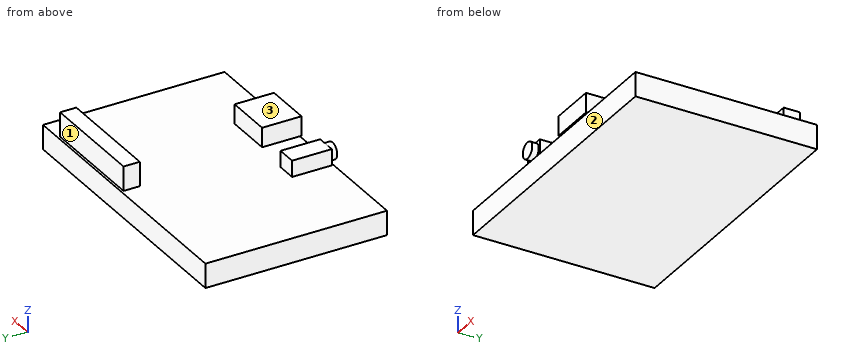
Autodesk Inventor part; units mm, degrees
ref_plane "YZ Plane" through (0, 0, 0) normal (1, 0, 0) x (0, 1, 0)
ref_plane "XZ Plane" through (0, 0, 0) normal (0, 1, 0) x (-1, 0, 0)
ref_plane "XY Plane" through (0, 0, 0) normal (0, 0, 1) x (1, 0, 0)
sketch "Sketch1" plane through (0, 0, 0) normal (0, 0, 1) x (1, 0, 0)
  line L0 (0, 0) -> (85.75, 0)
  line L1 (85.75, 0) -> (85.75, 56)
  line L2 (85.75, 56) -> (0, 56)
  line L3 (0, 56) -> (0, 0)
  dimension "d0" = 85.75
  dimension "d1" = 56
extrude "Extrusion1" add sketch "Sketch1" along normal blind 7.5
sketch "Sketch3" plane through (0, 0, 7.5) normal (0, 0, 1) x (1, 0, 0)
  line L0 (78, 55.25) -> (44.5, 55.25)
  line L1 (44.5, 55.25) -> (44.5, 50.25)
  line L2 (44.5, 50.25) -> (78, 50.25)
  line L3 (78, 50.25) -> (78, 55.25)
  line L4 (85.75, 56) -> (0, 56)
  line L5 (85.75, 0) -> (85.75, 56)
  point P0 (0, 0)
  dimension "d19" = 33.5
  dimension "d20" = 5
  dimension "d21" = 0.75
  dimension "d22" = 7.75
extrude "Extrusion3" add sketch "Sketch3" along normal blind 7.5
sketch "Sketch4" plane through (0, 0, 7.5) normal (0, 0, 1) x (1, 0, 0)
  line L0 (46, 11.65) -> (60.5, 11.65)
  line L1 (60.5, 11.65) -> (60.5, -0.5)
  line L2 (60.5, -0.5) -> (46, -0.5)
  line L3 (46, -0.5) -> (46, 11.65)
  line L4 (0, 0) -> (85.75, 0)
  line L5 (85.75, 0) -> (85.75, 56)
  dimension "d25" = 14.5
  dimension "d26" = 12.15
  dimension "d28" = 0.5
  dimension "d29" = 25.25
extrude "Extrusion4" add sketch "Sketch4" along normal blind 6
sketch "Sketch5" plane through (0, 0, 7.5) normal (0, 0, 1) x (1, 0, 0)
  line L0 (28.3, 12.75) -> (34.4, 12.75)
  line L1 (34.4, 12.75) -> (34.4, 0.5)
  line L2 (34.4, 0.5) -> (28.3, 0.5)
  line L3 (28.3, 0.5) -> (28.3, 12.75)
  line L4 (0, 0) -> (46, 0)
  line L5 (0, 56) -> (0, 0)
  dimension "d32" = 12.25
  dimension "d33" = 6.1
  dimension "d35" = 28.3
  dimension "d36" = 0.5
extrude "Extrusion5" add sketch "Sketch5" along normal blind 5
sketch "Sketch6" plane through (28.3, 0.5, 7.5) normal (0, -1, 0) x (1, 0, 0)
  line L0 (6.1, 5) -> (0, 5)
  line L1 (3.05, 5) -> (3.05, 2.5)
  circle A0 centre (3.05, 2.5) radius 2.5
  point P0 (-28.3, -7.5)
  dimension "d39" = 2.5
  dimension "d40" = 5
extrude "Extrusion6" add sketch "Sketch6" along normal blind 2
properties part number "RaspberryPi3_Screen"
Verification items for the finished model (mm, model axes). Face numbers are marked on the shaded views. A direction names the side the tool comes from. Coordinates: 2 decimals unless noted, no trailing zeros. Write each loop counter-clockwise with the first axis right and the second up, starting at its lowest first coordinate (ties: lowest second). Pieces come first, ordered by that corner, then holes. Notation, with made-up numbers: M -10.5,51.25 L 5.5,51.25 A21 cw 5.5,79.25 Z; hole C -2,38.5 d1. An arc over 180 degrees is marked long. Use a Markdown table: item, result.
Q1. Sectioned sample at A-A, the plane y = 3.5. Record the boundary of the cut face in (x, z).
Reply:
| item | result |
|---|---|
| outline | M 0,0 L 85.75,0 L 85.75,7.5 L 60.5,7.5 L 60.5,13.5 L 46,13.5 L 46,7.5 L 34.4,7.5 L 34.4,12.5 L 28.3,12.5 L 28.3,7.5 L 0,7.5 Z |
Q2. Sectioned sample at C-C, the plane z = 6.5. Record the boundary of the cut face in (x, y), plus the area to 3 significant figures.
Reply:
| item | result |
|---|---|
| outline | M 0,0 L 85.75,0 L 85.75,56 L 0,56 Z |
| area | 4,800 mm² |
Q3. Go/stop test with flat-tipped pins: P1, Ø5.5, axis at x = 30.5, z = 10.5, coming from the +Y side; P2, Ø2, axis at x = 54.5, z = 12, coming from the +Y side; P3, Ø2, axis at x = 55.5, y = 31, coming from the +Z side; P4, Ø8, axis at x = 76.5, y = 28, coming from the -Z side. Record where each tip stops, or that it passes through.
Reply:
| item | result |
|---|---|
| P1 | stops at y = 12.75 |
| P2 | stops at y = 55.25 |
| P3 | stops at z = 7.5 |
| P4 | stops at z = 0 |
Q4. Sectioned sample at B-B, the plane x = 57. Record the boundary of the cut face in (y, z), plus the area to 3 significant figures.
Reply:
| item | result |
|---|---|
| outline | M -0.5,7.5 L 0,7.5 L 0,0 L 56,0 L 56,7.5 L 55.25,7.5 L 55.25,15 L 50.25,15 L 50.25,7.5 L 11.65,7.5 L 11.65,13.5 L -0.5,13.5 Z |
| area | 530 mm² |
Q5. Set-up check for the marked faces 1, 2 and 3: record each of +Z, -Z, +X, -X, +Y, -Y from which the full face is reachable in a straight line by a thin tool's end or side.
Reply:
| item | result |
|---|---|
| face 1 | +Z, +X, -X, +Y |
| face 2 | -Z, +X, -X, -Y |
| face 3 | +Z, +X, -X, -Y |
Q6. Thickness scan on line 1 (Z direction, x = 78.5, y = 50.5); line 2 (Y direction, x = 48.5, z = 4.25); line 3 (Y direction, x = 31, z = 8.75). Record the ranges inside material, lowest first.
Reply:
| item | result |
|---|---|
| line 1 | z = 0 to 7.5 |
| line 2 | y = 0 to 56 |
| line 3 | y = -1.5 to 12.75 |
Q7. Sectioned sample at D-D, the plane x = 67. Record the boundary of the cut face in (y, z), plus the area to 4 significant figures.
Reply:
| item | result |
|---|---|
| outline | M 0,0 L 56,0 L 56,7.5 L 55.25,7.5 L 55.25,15 L 50.25,15 L 50.25,7.5 L 0,7.5 Z |
| area | 457.5 mm² |
